```python
from build123d import *

# Parameters (mm, degrees)
SKETCH_R           = 22.9254053499
PAD_DEPTH          = 40
SKETCH001_R        = 18.304244
POCKET_DEPTH       = 30
SKETCH002_R        = 5.45658
PAD001_DEPTH       = 2
SKETCH003_R        = 4.228884
PAD002_DEPTH       = 20
FILLET_R           = 1
SKETCH004_W        = 47.033489
SKETCH004_H        = 47.446069
PAD003_DEPTH       = 10
SKETCH005_W        = 6
SKETCH005_H        = 6
POCKET001_DEPTH    = 10
POLARPATTERN_COUNT = 3
SKETCH006_W        = 48.955269
SKETCH006_H        = 10.757687
POCKET002_DEPTH    = 47.447069
SKETCH007_W        = 8.584595
SKETCH007_H        = 2.239462
POCKET003_DEPTH    = 8


with BuildPart() as part:
    # Sketch → Pad (new body)
    with BuildSketch(Plane.XY):
        Circle(SKETCH_R)
    extrude(amount=PAD_DEPTH)

    # Sketch001 (on Face3 of Pad) → Pocket (cut)
    with BuildSketch(Plane.XY.offset(40)):
        Circle(SKETCH001_R)
    extrude(amount=-POCKET_DEPTH, mode=Mode.SUBTRACT)

    # Sketch002 (on Face5 of Pocket) → Pad001 (join)
    with BuildSketch(Plane.XY.offset(10)):
        Circle(SKETCH002_R)
    extrude(amount=PAD001_DEPTH)

    # Sketch003 (on Face7 of Pad001) → Pad002 (join)
    with BuildSketch(Plane.XY.offset(12)):
        Circle(SKETCH003_R)
    extrude(amount=PAD002_DEPTH)

    # Fillet
    fillet_edges = [part.edges().sort_by_distance(p)[0] for p in [
        (-4.228884, 0, 32),
    ]]
    fillet(fillet_edges, radius=FILLET_R)

    # Sketch004 (on Face8 of Fillet) → Pad003 (join)
    with BuildSketch(Plane.XY.offset(40)):
        with Locations((0.1454045, -0.1830035)):
            Rectangle(SKETCH004_W, SKETCH004_H)
    extrude(amount=PAD003_DEPTH)

    # Sketch005 (on Face6 of Pad003) → Pocket001 (cut)
    with BuildSketch(Plane.XZ.offset(23.906038)):
        with Locations((-0.0695171845, 4.0478014172)):
            Rectangle(SKETCH005_W, SKETCH005_H)
    pocket001 = extrude(amount=-POCKET001_DEPTH, mode=Mode.SUBTRACT)

    # PolarPattern: Pocket001 ×3 about axis
    polarpattern_axis = Axis((0, 0, 0), (0, 0, 1))
    for i in range(1, POLARPATTERN_COUNT):
        add(pocket001.rotate(polarpattern_axis, i * 360 / POLARPATTERN_COUNT), mode=Mode.SUBTRACT)

    # Sketch006 (on Face6 of PolarPattern) → Pocket002 (cut, through all)
    with BuildSketch(Plane.XZ.offset(23.906038)):
        with Locations((-0.0126055, 45.3770425)):
            Rectangle(SKETCH006_W, SKETCH006_H)
    extrude(amount=-POCKET002_DEPTH, mode=Mode.SUBTRACT)

    # Sketch007 (on Face2 of Pocket002) → Pocket003 (cut)
    with BuildSketch(Plane.XY.offset(39.998199)):
        with Locations((0.2128695, 20.199645)):
            Rectangle(SKETCH007_W, SKETCH007_H)
    extrude(amount=-POCKET003_DEPTH, mode=Mode.SUBTRACT)


solid = part.part
```
Source: CAD feature listing. Evaluate the final solid. Frame: model axes, mm. A direction names the side the tool comes from. Round coordinates to 2 decimals unless told otherwise and drop trailing zeros. Write each loop counter-clockwise with the first axis right and the second up, starting at its lowest first coordinate (ties: lowest second). Pieces come first, ordered by that corner, then holes. Notation, with made-up numbers: M 45,89 L 65,89 A22 ccw 65,125 Z; hole C 49,68.5 d9. An arc over 180 degrees is marked long. Answer as a JSON object with one key per item and string values. Group by question number.
(1) Section query D-D on y = -19. Output: boundary loops of the cut face in (x, z), then the cut area to 3 significant figures.
(2) Section query B-B on x = 0. Output: boundary loops of the cut face in (y, z), then the cut area to 3 significant figures.
(3) Reachability of faces 4 (the flat face through (-15.4, -10.3, 39.998)), 5 (the flat face through (0, 19.08, 36)), 6 (the flat face through (16, 9, 7.048)), 7 (the flat face through (0, -18, 7.048)) from +Z, -Z, +X, -X, +Y, -Y: full face, straight path, thin tool, end or side. Return the list, or none.
(4) Section query C-C on y = 0. Output: boundary loops of the cut face in (x, z), then the cut area to 3 significant figures.
(5) Ray query, line 1 (Y direction, x = 0, z = 29.25); line 2 (Z direction, x = 17, y = 9.5); line 3 (X direction, y = -1, z = 27.5). Return the intervals inside material, ascending. Write a range as [from, to].
(6) Mould query, pull axis X, two halves, no side actions, for faces 1 (the flat face through (-3.07, -18, 4)), 2 (the flat face through (0, 0, 0)), 3 (the flat face through (4.505, 20, 36)). Classes: +X half, -X half, draft (parallel to the pull), parting line (faces both ways), or undercut.
(7) First-contact query: pin 1 (10 mm diameter, centred on x = -6.5, z = 9, fed in from -Y); pin 2 (5 mm diameter, centred on x = -16.5, z = 20, fed in from -Y); pin 3 (3.5 mm diameter, centred on x = 1.5, y = 0.5, fed in from +Z); pin 4 (6 mm diameter, centred on y = -2.5, z = 11.5, fed in from -X). Flat tips, straight axial feed; report the tip coordinate or a pass-through.
(8) Section query A-A on z = 30. Output: boundary loops of the cut face in (x, y).
Computed values:
{
 "1": {"outline": "M -12.83,0 L 12.83,0 L 12.83,40 L -12.83,40 Z; hole M -3.07,1.05 L 2.93,1.05 L 2.93,7.05 L -3.07,7.05 Z", "area": "990 mm^2"},
 "2": {"outline": "M -22.93,0 L 22.93,0 L 22.93,40 L 21.32,40 L 21.32,32 L 19.08,32 L 19.08,40 L 18.3,40 L 18.3,10 L 5.46,10 L 5.46,12 L 4.23,12 L 4.23,31 A1 ccw 3.23,32 L -3.23,32 A1 ccw -4.23,31 L -4.23,12 L -5.46,12 L -5.46,10 L -18.3,10 L -18.3,40 L -22.93,40 L -22.93,7.05 L -13.91,7.05 L -13.91,1.05 L -22.93,1.05 Z", "area": "854 mm^2"},
 "3": {"face 4": "+Z, +X, -X, +Y, -Y", "face 5": "+Z", "face 6": "none", "face 7": "-Y"},
 "4": {"outline": "M -22.93,0 L 22.93,0 L 22.93,40 L 18.3,40 L 18.3,10 L 5.46,10 L 5.46,12 L 4.23,12 L 4.23,31 A1 ccw 3.23,32 L -3.23,32 A1 ccw -4.23,31 L -4.23,12 L -5.46,12 L -5.46,10 L -18.3,10 L -18.3,40 L -22.93,40 Z", "area": "926 mm^2"},
 "5": {"line 1": "[-22.93, -18.3], [-4.23, 4.23], [18.3, 22.93]", "line 2": "[0, 1.05], [7.05, 40]", "line 3": "[-22.9, -18.28], [-4.11, 4.11], [18.28, 22.9]"},
 "6": {"face 1": "undercut", "face 2": "draft", "face 3": "undercut"},
 "7": {"pin 1": "y = -22.88", "pin 2": "y = -18.15", "pin 3": "z = 32", "pin 4": "x = -22.93"},
 "8": {"outline": "C 0,0 d45.85; C 0,0 d8.46; hole C 0,0 d36.61"}
}
